from build123d import *

# Parameters (mm, degrees)
F0_W     = 34
F0_H     = 30
F1_DEPTH = 25.4
F2_R     = 4
F3_DEPTH = 30.001
F4_W     = 17.084244
F4_H     = 30
F5_DEPTH = 6.35


with BuildPart() as f1:
    # F0 (on Top) → F1 (new body)
    with BuildSketch(Plane.XY):
        Rectangle(F0_W, F0_H)
    extrude(amount=F1_DEPTH)

    # F2 (on face) → F3 (cut, through all)
    with BuildSketch(Plane.XZ.offset(15)):
        with Locations((0, 10.498762)):
            Circle(F2_R)
    extrude(amount=-F3_DEPTH, mode=Mode.SUBTRACT)

    # F4 (on face) → F5 (cut)
    with BuildSketch(Plane.XY.offset(25.4)):
        Rectangle(F4_W, F4_H)
    extrude(amount=-F5_DEPTH, mode=Mode.SUBTRACT)


solid = f1.part
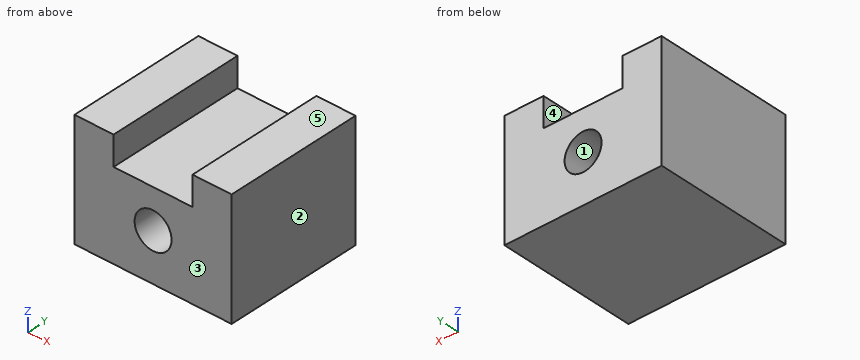
Model file for the job. Use its own axes, mm. Face numbers are marked on the shaded views. A direction names the side the tool comes from. Coordinates: 2 decimals unless noted, no trailing zeros. Write each loop counter-clockwise with the first axis right and the second up, starting at its lowest first coordinate (ties: lowest second). Pieces come first, ordered by that corner, then holes. Notation, with made-up numbers: (62, 40.25) -> (67, 40.25) arc R11 cw to (67, 51.25) -> close; hole circle Ø11 at (-10.75, -5.75). An arc over 180 degrees is marked (long way). One line per item, written item: value. Start each with the question number.
1) Slice it at D-D on x = 8. Write the cut outline in (y, z).
2) Pull direction X, two halves, no side cores. Call the marked faces 1, 2 and 3: +X half, -X half, draft (parallel to the pull), parting line (faces both ways), or undercut.
3) Slice it at A-A on x = 0. Write the cut outline in (y, z).
4) Which spindle directions (+Z, -Z, +X, -X, +Y, -Y) get a long thin tool onto all of the face, cutting with end or side? Do the marked faces 4 and 5. Say none if no direction does.
5) Slice it at C-C on y = 1.5. Write the cut outline in (x, z), then the cut area to 3 significant figures.
6) Probe probe 1 along Z at (x, y) = (0, 4); probe 2 along X at (y, z) = (13, 20.5); probe 3 along Z at (x, y) = (-6, -3). List the from-to ranges inside material, lowest first.
7) Slice it at B-B on z = 21.5. Write the cut outline in (x, y), then the cut area to 3 significant figures.
8) Flat gauge pins, fed straight in: pin 1 Ø2 at (x, z) = (0.5, 12.5) entering from +Y; pin 2 Ø5 at (x, y) = (3.5, -2) entering from +Z. Where does each tip first touch, or does it go through?
Answers follow:
1. outline: (-15, 0) -> (15, 0) -> (15, 19.05) -> (-15, 19.05) -> close
2. face 1: undercut
2. face 2: +X half
2. face 3: draft
3. outline: (-15, 0) -> (15, 0) -> (15, 6.5) -> (-15, 6.5) -> close; (-15, 14.5) -> (15, 14.5) -> (15, 19.05) -> (-15, 19.05) -> close
4. face 4: +Z, +Y, -Y
4. face 5: +Z, +X, -X, +Y, -Y
5. outline: (-17, 0) -> (17, 0) -> (17, 25.4) -> (8.54, 25.4) -> (8.54, 19.05) -> (-8.54, 19.05) -> (-8.54, 25.4) -> (-17, 25.4) -> close; hole circle Ø8 at (0, 10.5)
5. area: 705 mm2
6. probe 1: 0 to 6.5, 14.5 to 19.05
6. probe 2: -17 to -8.54, 8.54 to 17
6. probe 3: 0 to 19.05
7. outline: (-17, -15) -> (-8.54, -15) -> (-8.54, 15) -> (-17, 15) -> close; (8.54, -15) -> (17, -15) -> (17, 15) -> (8.54, 15) -> close
7. area: 507 mm2
8. pin 1: through
8. pin 2: z = 19.05
